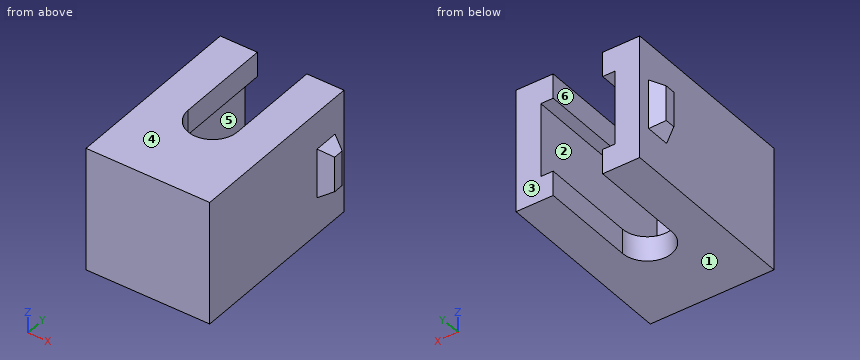
Autodesk Inventor part; units mm, degrees
ref_plane "YZ Plane" through (0, 0, 0) normal (1, 0, 0) x (0, 1, 0)
ref_plane "XZ Plane" through (0, 0, 0) normal (0, 1, 0) x (-1, 0, 0)
ref_plane "XY Plane" through (0, 0, 0) normal (0, 0, 1) x (1, 0, 0)
sketch "Sketch1" plane through (0, 0, 0) normal (0, 1, 0) x (-1, 0, 0)
  line L0 (-2.5, 2.5) -> (2.5, 2.5)
  line L1 (2.5, 2.5) -> (2.5, -2.5)
  line L2 (2.5, -2.5) -> (-2.5, -2.5)
  line L3 (-2.5, -2.5) -> (-2.5, 2.5)
  line L4 (-2.5, 2.5) -> (2.5, -2.5) construction
  line L5 (2.5, 2.5) -> (-2.5, -2.5) construction
  point P0 (0, 0)
  dimension "d0" = 5
  dimension "d1" = 5
extrude "Extrusion1" add sketch "Sketch1" along normal blind 7.5
shell "Shell1" thickness 1 removed faces 1 at (-0.8333, 7.5, -0.8333)
sketch "Sketch4" plane through (0, 7.5, 0) normal (0, 1, 0) x (1, 0, 0)
  point P0 (0, 0)
sketch "Sketch5" plane through (0, 7.5, 0) normal (0, 1, 0) x (1, 0, 0)
  point P0 (0, 0)
sketch "Sketch6" plane through (0, 7.5, 0) normal (0, 1, 0) x (1, 0, 0)
  point P0 (0, 0)
sketch "Sketch7" plane through (0, 0, 0) normal (0, -1, 0) x (1, 0, 0)
  point P0 (0, 0)
sketch "Sketch8" plane through (-2.5, 0, -2.5) normal (-1, 0, 0) x (0, 0, 1)
  point P0 (2.5, 0)
sketch "Sketch9" plane through (2.5, 0, 2.5) normal (1, 0, 0) x (0, 0, -1)
  line L0 (1.5, 6) -> (3.5, 6)
  line L1 (3.5, 6) -> (3.5, 7)
  line L2 (3.5, 7) -> (1.5, 7)
  line L3 (1.5, 7) -> (1.5, 6)
  line L4 (1.5, 6) -> (3.5, 7) construction
  line L5 (3.5, 6) -> (1.5, 7) construction
  line L6 (0, 7.5) -> (5, 7.5)
  point P0 (2.5, 0)
  point P1 (2.5, 6.5)
  dimension "d10" = 1
  dimension "d14" = 2
  dimension "d15" = 1
extrude "Extrusion4" add sketch "Sketch9" along normal blind 0.5 draft -30
sketch "Sketch10" plane through (-2.5, 0, -2.5) normal (-1, 0, 0) x (0, 0, 1)
  line L0 (1.5, 6) -> (3.5, 6)
  line L1 (3.5, 6) -> (3.5, 7)
  line L2 (3.5, 7) -> (1.5, 7)
  line L3 (1.5, 7) -> (1.5, 6)
  line L4 (1.5, 6) -> (3.5, 7) construction
  line L5 (3.5, 6) -> (1.5, 7) construction
  line L6 (0, 7.5) -> (5, 7.5)
  point P0 (2.5, 0)
  point P1 (2.5, 6.5)
  dimension "d13" = 1
  dimension "d16" = 2
  dimension "d17" = 1
extrude "Extrusion5" add sketch "Sketch10" along normal blind 0.5 draft -30
sketch "Sketch11" plane through (2.5, 0, -2.5) normal (0, 0, -1) x (-1, 0, 0)
  line L0 (2.5, 7.862) -> (2.5, 3.6245) construction
  line L1 (1.5, 7.862) -> (1.5, 3.6245)
  line L2 (3.5, 3.6245) -> (3.5, 7.862)
  arc A0 (3.5, 7.862) -> (1.5, 7.862) centre (2.5, 7.862) ccw
  arc A1 (1.5, 3.6245) -> (3.5, 3.6245) centre (2.5, 3.6245) ccw
  point P0 (2.5, 0)
  point P1 (2.5, 5.7432)
  dimension "d20" = 2
extrude "Extrusion6" cut sketch "Sketch11" against normal through all
equation "\"d16\" = d14"
equation "\"d17\" = d15"
properties part number "snapfit_v11"
Could you check a few things on this model? Use its own coordinates, in mm. Face numbers are marked on the shaded views. A direction names the side the tool comes from. Coordinates: 2 decimals unless noted, no trailing zeros. Write each loop counter-clockwise with the first axis right and the second up, starting at its lowest first coordinate (ties: lowest second). Pieces come first, ordered by that corner, then holes. Notation, with made-up numbers: (-37, -9.75) - (-18, -9.75) arc R23 cw to (-18, 18.25) - close; hole circle Ø9 at (83.5, -26.5). An arc over 180 degrees is marked (long way). Use a Markdown table: item, result.
Q1. I'm going to push flat-ended pins straight in: pin 1 Ø1 at (x, z) = (0, 0.5) entering from +Y; pin 2 Ø0.8 at (y, z) = (5.5, -2) entering from +X; pin 3 Ø0.8 at (y, z) = (6.5, -2) entering from -X. Where does each tip first touch, or does it pass through?
Geometry check:
| item | result |
|---|---|
| pin 1 | stops at y = 1 |
| pin 2 | stops at x = 2.5 |
| pin 3 | stops at x = -2.5 |
Q2. Thinking about a two-plate mould opening in Z: for the marked faces 1, 2 and 3, which applies, +Z half, -Z half, draft (parallel to the pull), parting line (faces both ways), or undercut?
Geometry check:
| item | result |
|---|---|
| face 1 | -Z half |
| face 2 | undercut |
| face 3 | draft |
Q3. Imagine slicing it at B-B (y = 1.75). List the corners of the cut face in (x, z) for me.
Geometry check:
| item | result |
|---|---|
| outline | (-2.5, -2.5) - (2.5, -2.5) - (2.5, 2.5) - (-2.5, 2.5) - close; hole (-1.5, -1.5) - (1.5, -1.5) - (1.5, 1.5) - (-1.5, 1.5) - close |
Q4. Which directions (+Z, -Z, +X, -X, +Y, -Y) give clear straight access to the entire face, cutting with the end or side of a thin tool? Please do the marked faces 4, 5 and 6.
Geometry check:
| item | result |
|---|---|
| face 4 | +Z, +X, -X, +Y, -Y |
| face 5 | +Y |
| face 6 | +Z, -Z, +Y |
Q5. Imagine slicing it at C-C (z = 1.15). List the corners of the cut face in (x, y) for me, and give its area (3 significant figures).
Geometry check:
| item | result |
|---|---|
| outline | (-2.5, 0) - (2.5, 0) - (2.5, 7.5) - (1.5, 7.5) - (1.5, 1) - (-1.5, 1) - (-1.5, 7.5) - (-2.5, 7.5) - close |
| area | 18.0 mm2 |
Q6. Imagine slicing it at A-A (y = 6.5). List the corners of the cut face in (x, z) for me, and give its area (3 significant figures).
Geometry check:
| item | result |
|---|---|
| outline | (-3, -0.71) - (-2.5, -1) - (-2.5, -2.5) - (-1, -2.5) - (-1, -1.5) - (-1.5, -1.5) - (-1.5, 1.5) - (-1, 1.5) - (-1, 2.5) - (-2.5, 2.5) - (-2.5, 1) - (-3, 0.71) - close; (1, -2.5) - (2.5, -2.5) - (2.5, -1) - (3, -0.71) - (3, 0.71) - (2.5, 1) - (2.5, 2.5) - (1, 2.5) - (1, 1.5) - (1.5, 1.5) - (1.5, -1.5) - (1, -1.5) - close |
| area | 13.7 mm2 |
Q7. Please list where these lines run through material, in increasing order: L1, parallel to X at y = 3.25, z = -1.4; L2, parallel to X at y = 7.25, z = -1.9.
Geometry check:
| item | result |
|---|---|
| L1 | x = -2.5 to -1.5, 1.5 to 2.5 |
| L2 | x = -2.5 to -1, 1 to 2.5 |
Q8. Imagine slicing it at D-D (x = 0). List the corners of the cut face in (y, z) for me.
Geometry check:
| item | result |
|---|---|
| outline | (0, -2.5) - (2.62, -2.5) - (2.62, -1.5) - (1, -1.5) - (1, 1.5) - (2.62, 1.5) - (2.62, 2.5) - (0, 2.5) - close |
